from build123d import *

# Parameters (mm, degrees)
F1_DEPTH = 849.122
F3_DEPTH = 23.877


with BuildPart() as f1:
    # F0 (on Front) → F1 (new body, symmetric)
    with BuildSketch(Plane.XZ):
        with BuildLine():
            Line((63.246, 11.938), (-63.246, 11.938))
            ThreePointArc((-63.246, 11.938), (-66.658497, 10.524497), (-68.072, 7.112))
            Line((-68.072, 7.112), (-68.072, -7.112))
            ThreePointArc((-68.072, -7.112), (-66.658497, -10.524497), (-63.246, -11.938))
            Line((-63.246, -11.938), (63.246, -11.938))
            ThreePointArc((63.246, -11.938), (66.658497, -10.524497), (68.072, -7.112))
            Line((68.072, -7.112), (68.072, 7.112))
            ThreePointArc((68.072, 7.112), (66.658497, 10.524497), (63.246, 11.938))
        make_face()
    extrude(amount=F1_DEPTH, both=True)

    # F2 (on face) → F3 (cut, through all)
    with BuildSketch(Plane.XY.offset(11.938)):
        Polygon((-68.072, -849.122), (68.072, -849.122), (-68.072, -712.978), align=None)
        Polygon((68.072, 849.122), (-68.072, 849.122), (68.072, 712.978), align=None)
    extrude(amount=-F3_DEPTH, mode=Mode.SUBTRACT)


solid = f1.part
For this review, take the finished solid that the model builds, in its own axes (mm). Give positions to 0.01 mm unless a question says otherwise; leave off trailing zeros. Loops run counter-clockwise (first coordinate to the right, second up) from the corner with the lowest first, then second, coordinate; pieces in that order, holes last. Notation, with made-up numbers: (-27, 61) -> (21, 61) arc R30 ccw to (21, 93) -> close; hole circle Ø5 at (27.25, 42.5). An arc over 180 degrees is marked (long way). One line per question, with ' | ' between items.
1) To check wall thickness, follow probe 1 along X at (y, z) = (-171.5, 7.5); probe 2 along X at (y, z) = (645.5, -8); probe 3 along Y at (x, z) = (-6, 0.25). State the ranges of each line that lie inside material, in increasing order.
Resolved:
probe 1: x = -68.06 to 68.06 | probe 2: x = -67.99 to 67.99 | probe 3: y = -775.05 to 787.05
2) We need section B-B (z = 1). Write out the cut boundary in (x, y), plus the area to 3 significant figures.
Resolved:
outline: (-68.07, -712.98) -> (68.07, -849.12) -> (68.07, 712.98) -> (-68.07, 849.12) -> close | area: 213,000 mm2
3) Insertion check: pin 1 Ø10 at (x, z) = (52.5, -6) entering from -Y; pin 2 Ø3 at (x, z) = (-18.5, -8.5) entering from -Y. Each pin has a flat end and moves straight along its axis. Give the tip position at first contact, or say it passes through.
Resolved:
pin 1: stops at y = -838.55 | pin 2: stops at y = -764.05
4) We need section A-A (x = 47). Write out the cut boundary in (y, z), plus the area to 3 significant figures.
Resolved:
outline: (-828.05, -11.94) -> (734.05, -11.94) -> (734.05, 11.94) -> (-828.05, 11.94) -> close | area: 37,300 mm2
